Geometry: final body of the model. Coordinates: model frame, mm. A direction names the side the tool comes from. Coordinates: 2 decimals unless noted, no trailing zeros. Order: outer loops, then holes, each group sorted by start corner. A loop starts at its lowest first (then second) coordinate and runs counter-clockwise, first axis right, second up. Notation, with made-up numbers: (73.5, 45) - (129.5, 45) arc R33 ccw to (129.5, 78) - close; hole circle Ø2 at (-27, 8). An arc over 180 degrees is marked (long way). Use a Markdown table: item, result. Add a question column.
```python
from build123d import *

# Parameters (mm, degrees)
F0_R     = 140
F0_R_2   = 113
F1_DEPTH = 2
F2_R     = 115
F2_R_2   = 113
F3_DEPTH = 60
F5_DEPTH = 2.001


with BuildPart() as f1:
    # F0 (on Top) → F1 (new body)
    with BuildSketch(Plane.XY):
        Circle(F0_R)
        Circle(F0_R_2, mode=Mode.SUBTRACT)
    extrude(amount=F1_DEPTH)

    # F2 (on face) → F3 (join)
    with BuildSketch(Plane.XY.offset(2)):
        Circle(F2_R)
        Circle(F2_R_2, mode=Mode.SUBTRACT)
    extrude(amount=F3_DEPTH)

    # F4 (on face) → F5 (cut, through all)
    with BuildSketch(Plane.XY.offset(2)):
        with BuildLine():
            ThreePointArc((-4.5, 129.5), (0, 125), (4.5, 129.5))
            Line((4.5, 129.5), (4.5, 139.9276598818))
            ThreePointArc((4.5, 139.9276598818), (2.2502907086, 139.9819138022), (0, 140))
            ThreePointArc((0, 140), (-2.2502907086, 139.9819138022), (-4.5, 139.9276598818))
            Line((-4.5, 139.9276598818), (-4.5, 129.5))
        make_face()
        with BuildLine():
            ThreePointArc((102.9190976917, 94.9086894353), (99.8151721136, 98.1678736448), (96.6080873732, 101.3256011781))
            Line((96.6080873732, 101.3256011781), (89.6990082559, 94.4165220608))
            ThreePointArc((89.6990082559, 94.4165220608), (89.6990082559, 88.0525610302), (96.0629692866, 88.0525610302))
            Line((96.0629692866, 88.0525610302), (102.9190976917, 94.9086894353))
        make_face()
        with BuildLine():
            ThreePointArc((140, 0), (139.9919631357, 1.500085806), (139.9678534654, 2.9999993836))
            Line((139.9678534654, 2.9999993836), (131.5000006164, 2.9999993836))
            ThreePointArc((131.5000006164, 2.9999993836), (127.0000006164, -1.5000006164), (131.5000006164, -6.0000006164))
            Line((131.5000006164, -6.0000006164), (139.8713694528, -6.0000006164))
            ThreePointArc((139.8713694528, -6.0000006164), (139.9678386691, -3.000689638), (140, 0))
        make_face()
        with BuildLine():
            ThreePointArc((95.1684959742, -102.6789042307), (98.41976806, -99.5668079985), (101.5693267645, -96.3518129596))
            Line((101.5693267645, -96.3518129596), (96.4165226772, -91.1990088723))
            ThreePointArc((96.4165226772, -91.1990088723), (90.0525616465, -91.1990088723), (90.0525616465, -97.562969903))
            Line((90.0525616465, -97.562969903), (95.1684959742, -102.6789042306))
        make_face()
        with BuildLine():
            Line((-4, -133.0000012327), (-4, -139.9428454763))
            ThreePointArc((-4, -139.9428454763), (0.5002584944, -139.9991062166), (5, -139.9106857963))
            Line((5, -139.9106857963), (5, -133.0000012327))
            ThreePointArc((5, -133.0000012327), (0.5, -128.5000012327), (-4, -133.0000012327))
        make_face()
        with BuildLine():
            Line((-95.5629692866, -91.5525622629), (-100.97984248, -96.9694354563))
            ThreePointArc((-100.97984248, -96.9694354563), (-97.8105621043, -100.1653330292), (-94.5401870301, -103.2577020677))
            Line((-94.5401870301, -103.2577020677), (-89.1990082559, -97.9165232936))
            ThreePointArc((-89.1990082559, -97.9165232936), (-89.1990082559, -91.5525622629), (-95.5629692866, -91.5525622629))
        make_face()
        with BuildLine():
            Line((-131.0000006164, 2.4999993836), (-139.9776768027, 2.4999993836))
            ThreePointArc((-139.9776768027, 2.4999993836), (-139.9856987687, -2.0010347926), (-139.8490257098, -6.5000006164))
            Line((-139.8490257098, -6.5000006164), (-131.0000006164, -6.5000006164))
            ThreePointArc((-131.0000006164, -6.5000006164), (-126.5000006164, -2.0000006164), (-131.0000006164, 2.4999993836))
        make_face()
        with BuildLine():
            Line((-89.5525616465, 94.0629686703), (-96.7140546298, 101.2244616536))
            ThreePointArc((-96.7140546298, 101.2244616536), (-99.9178627776, 98.063350432), (-103.01840372, 94.8008886824))
            Line((-103.01840372, 94.8008886824), (-95.9165226772, 87.6990076396))
            ThreePointArc((-95.9165226772, 87.6990076396), (-89.5525616465, 87.6990076396), (-89.5525616465, 94.0629686703))
        make_face()
    extrude(amount=-F5_DEPTH, mode=Mode.SUBTRACT)


solid = f1.part
```
1) Draft query along X for faces 3 (the cylindrical face through (-128.907, -54.617, 0.986)), 4 (the flat face through (-99.52, 91.3, 1.01)), 5 (the cylindrical face through (-89.13, -91.623, 1.014)), 6 (the flat face through (-94, 63, 0)). Return one class per face: released by +X, released by -X, zero draft, split by the parting line, or undercut.
2) Section query C-C (z = 9). Return the cut outline in (x, y).
3) Line query: line 1 (Y direction, x = 0, z = 42); line 2 (X direction, y = -58, z = 56.5); line 3 (Z direction, x = 62.5, y = -115). Output: solid intervals per line, ascending. Write a range as from..to.
4) First-contact query: pin 1 (1 mm diameter, centred on x = -11, z = 9.5, fed in from -Y); pin 2 (12 mm diameter, centred on y = -84.5, z = 42, fed in from +X); pin 3 (4 mm diameter, centred on y = 54.5, z = 49.5, fed in from -X). Flat tips, straight axial feed; report the tip coordinate or a pass-through.
5) Access query for faces 1 (the flat face through (-11, 115, 2)), 2 (the cylindrical face through (130.111, 51.684, 0.986)). Directions: +Z, -Z, +X, -X, +Y, -Y. A direction counts if a zero-diameter tool reaches every point of the face in a straight line with its end or side. Return the directions, or none.
6) Section query A-A (y = -60). Return the cut outline in (x, z), and give its area (3 significant figures).
7) Section query B-B (x = 0). Return the cut outline in (y, z).
From the geometry:
| question | item | result |
|---|---|---|
| 1 | face 3 | released by -X |
| 1 | face 4 | undercut |
| 1 | face 5 | undercut |
| 1 | face 6 | zero draft |
| 2 | outline | circle Ø230 at (0, 0); hole circle Ø226 at (0, 0) |
| 3 | line 1 | y = -115..-113, 113..115 |
| 3 | line 2 | x = -99.3..-96.98, 96.98..99.3 |
| 3 | line 3 | z = 0..2 |
| 4 | pin 1 | stops at y = -114.52 |
| 4 | pin 2 | stops at x = 84.04 |
| 4 | pin 3 | stops at x = -102.32 |
| 5 | face 1 | +Z |
| 5 | face 2 | +Z, -Z, +X, +Y |
| 6 | outline | (-126.49, 0) - (-95.75, 0) - (-95.75, 62) - (-98.11, 62) - (-98.11, 2) - (-126.49, 2) - close; (95.75, 0) - (126.49, 0) - (126.49, 2) - (98.11, 2) - (98.11, 62) - (95.75, 62) - close |
| 6 | area | 405 mm^2 |
| 7 | outline | (-128.53, 0) - (-113, 0) - (-113, 62) - (-115, 62) - (-115, 2) - (-128.53, 2) - close; (113, 0) - (125, 0) - (125, 2) - (115, 2) - (115, 62) - (113, 62) - close |
